Geometry: final body of the model. Coordinates: model frame, mm. Face numbers are marked on the shaded views. A direction names the side the tool comes from. Give positions to 0.01 mm unless a question says otherwise; leave off trailing zeros. Order: outer loops, then holes, each group sorted by start corner. A loop starts at its lowest first (then second) coordinate and runs counter-clockwise, first axis right, second up. Notation, with made-up numbers: (85, 73) -> (134, 73) arc R28 cw to (134, 98) -> close; hole circle Ø8 at (-28.5, 88). An arc over 180 degrees is marked (long way). Answer in a Markdown table with one row per item. Add a question column.
Q1. Cut plane D-D on x = 15.5. Return the cut outline in (y, z), and give its area (3 significant figures).
Q2. Cut plane A-A on z = -38.1. Return the cut outline in (x, y).
Q3. Line query: line 1 along X through (y, z) = (7.5, -38.1); line 2 along X through (y, z) = (51.5, -63). Output: solid intervals per line, ascending. Write a range as from..to.
Q4. Set-up query: the marked faces 1, 2 and 3. Return all of +Z, -Z, +X, -X, +Y, -Y with unobstructed straight access to the full face (end or side cutting, diameter ignored); none if empty.
Q5. Cut plane C-C on z = -68. Return the cut outline in (x, y).
Q6. Contact query for flat-ended pins moving along their axis: P1, Ø4, axis at y = 8.5, z = -22.5, coming from the +X side; P2, Ø25, axis at x = 46.482, z = -38.1, coming from the +Y side; P3, Ø2, axis at y = 55.5, z = -67.5, coming from the +X side. Output: stop coordinate, or through.
Q7. Cut plane B-B on x = 103. Return the cut outline in (y, z), and give its area (3 significant figures).
Q8. Pull-direction query (Z, two-part tool) for the marked faces 4, 5 and 6; classes: +Z half, -Z half, draft (parallel to the pull), parting line (faces both ways), or undercut.
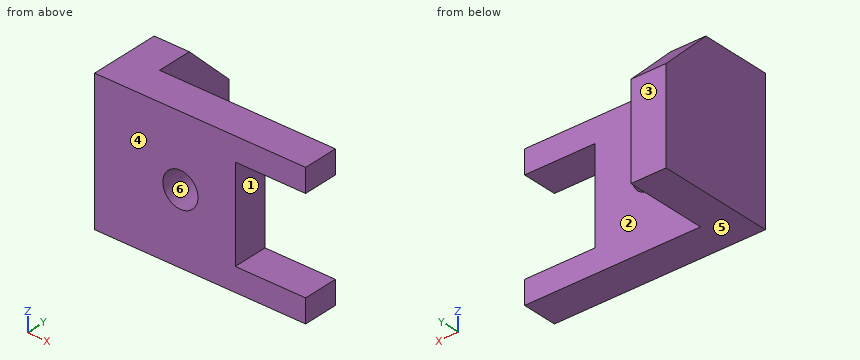
Autodesk Inventor part; units mm, degrees
ref_plane "YZ Plane" through (0, 0, 0) normal (1, 0, 0) x (0, 1, 0)
ref_plane "XZ Plane" through (0, 0, 0) normal (0, 1, 0) x (-1, 0, 0)
ref_plane "XY Plane" through (0, 0, 0) normal (0, 0, 1) x (1, 0, 0)
sketch "Sketch1" plane through (0, 0, 0) normal (0, 0, 1) x (1, 0, 0)
  line L0 (0, 0) -> (114.3, 0)
  line L1 (0, 0) -> (0, 63.5)
  line L2 (0, 63.5) -> (19.05, 63.5)
  line L3 (114.3, 0) -> (114.3, 19.05)
  line L4 (114.3, 19.05) -> (19.05, 19.05)
  line L5 (19.05, 19.05) -> (19.05, 63.5)
  dimension "d0" = 114.3
  dimension "d1" = 63.5
  dimension "d2" = 19.05
  dimension "d3" = 19.05
extrude "Extrusion1" add sketch "Sketch1" against normal blind 76.2
sketch "Sketch2" plane through (19.05, 19.05, 0) normal (1, 0, 0) x (0, 0, -1)
  line L0 (76.2, -19.05) -> (76.2, 44.45)
  line L1 (0, 44.45) -> (76.2, 44.45)
  line L2 (25.4, 44.45) -> (0, 44.45)
  line L3 (0, 44.45) -> (0, 19.05)
  line L4 (0, 44.45) -> (0, -19.05)
  line L5 (0, 19.05) -> (25.4, 44.45)
  dimension "d7" = 25.4
extrude "Extrusion2" cut sketch "Sketch2" against normal through all
sketch "Sketch3" plane through (114.3, 0, 0) normal (1, 0, 0) x (0, 0, -1)
  line L0 (12.7, 19.05) -> (12.7, 0)
  line L1 (0, 0) -> (76.2, 0)
  line L2 (12.7, 19.05) -> (63.5, 19.05)
  line L3 (0, 19.05) -> (76.2, 19.05)
  line L4 (63.5, 19.05) -> (63.5, 0)
  line L5 (12.7, 0) -> (63.5, 0)
  dimension "d11" = 50.8
extrude "Extrusion3" cut sketch "Sketch3" against normal blind 38.1
sketch "Sketch4" plane through (19.05, 19.05, 0) normal (0, 1, 0) x (1, 0, 0)
  line L0 (95.25, 0) -> (0, 0)
  line L1 (95.25, 0) -> (95.25, 12.7)
  point P0 (-19.05, 0)
  point P1 (27.432, 38.1)
  dimension "d14" = 38.1
  dimension "d15" = 67.818
hole "Hole1" at (46.482, 19.05, -38.1) direction (0, -1, 0) diameter 19.05 end through all
properties part number "Assignment 3.6 - L-Bracket"
Completed:
| question | item | result |
|---|---|---|
| 1 | outline | (0, -76.2) -> (63.5, -76.2) -> (63.5, -25.4) -> (38.1, 0) -> (0, 0) -> close |
| 1 | area | 4,520 mm² |
| 2 | outline | (0, 0) -> (36.96, 0) -> (36.96, 19.05) -> (19.05, 19.05) -> (19.05, 63.5) -> (0, 63.5) -> close; (56.01, 0) -> (76.2, 0) -> (76.2, 19.05) -> (56.01, 19.05) -> close |
| 3 | line 1 | x = 0..36.96, 56.01..76.2 |
| 3 | line 2 | x = 0..19.05 |
| 4 | face 1 | +X, +Y, -Y |
| 4 | face 2 | +Z, -Z, +X, +Y |
| 4 | face 3 | +Z, -Z, +X, -X, +Y |
| 5 | outline | (0, 0) -> (114.3, 0) -> (114.3, 19.05) -> (19.05, 19.05) -> (19.05, 63.5) -> (0, 63.5) -> close |
| 6 | P1 | stops at x = 76.2 |
| 6 | P2 | stops at y = 19.05 |
| 6 | P3 | stops at x = 19.05 |
| 7 | outline | (0, -76.2) -> (19.05, -76.2) -> (19.05, -63.5) -> (0, -63.5) -> close; (0, -12.7) -> (19.05, -12.7) -> (19.05, 0) -> (0, 0) -> close |
| 7 | area | 484 mm² |
| 8 | face 4 | draft |
| 8 | face 5 | -Z half |
| 8 | face 6 | undercut |
